Build history of the part. All positions in model axes, mm. A direction names the side the tool comes from. Coordinates: 2 decimals unless noted, no trailing zeros. Order: outer loops, then holes, each group sorted by start corner. A loop starts at its lowest first (then second) coordinate and runs counter-clockwise, first axis right, second up. Notation, with made-up numbers: (12.25, -17.5) - (26.25, -17.5) arc R17 cw to (26.25, 3.5) - close; hole circle Ø7 at (39.25, -26.5). An arc over 180 degrees is marked (long way). One line per item, written item: value.
from build123d import *

# Parameters (mm, degrees)
F1_START = -5
F1_DEPTH = 5
F2_DEPTH = 5
F3_DEPTH = 10
F4_DEPTH = 5
F5_DEPTH = 5


# Not quite as in the source:
# - after a boolean that leaves OpenCascade's solid faulty, fix() repairs it
# - a feature names something its author has since deleted; it is built from what else it names


with BuildPart() as f1:
    # F0 (on Top) → F1 (new body)
    with BuildSketch(Plane.XY.offset(F1_START)):
        with BuildLine():
            Line((0, 12), (-48.538644398, 12))
            Line((-48.538644398, 12), (-53.6749476013, 12))
            Line((-53.6749476013, 12), (-57.7667724561, 12))
            Line((-57.7667724561, 12), (-67.9485099174, 12))
            ThreePointArc((-67.9485099174, 12), (-68.6421053306, 7.0186448683), (-68.9710084021, 2))
            Line((-68.9710084021, 2), (0, 2))
            Line((0, 2), (0, 12))
        make_face()
        with BuildLine():
            Line((0, -7), (0, -2))
            Line((0, -2), (-68.9710084021, -2))
            ThreePointArc((-68.9710084021, -2), (-68.8529103806, -4.5029692558), (-68.6440092069, -7))
            Line((-68.6440092069, -7), (-58.5832740635, -7))
            Line((-58.5832740635, -7), (-54.5527267879, -7))
            Line((-54.5527267879, -7), (-49.5075751779, -7))
            Line((-49.5075751779, -7), (0, -7))
        make_face()
        with BuildLine():
            Line((68.9710084021, -2), (0, -2))
            Line((0, -2), (0, -7))
            Line((0, -7), (49.5075751779, -7))
            Line((49.5075751779, -7), (54.5527267879, -7))
            Line((54.5527267879, -7), (58.5832740635, -7))
            Line((58.5832740635, -7), (68.6440092069, -7))
            ThreePointArc((68.6440092069, -7), (68.8529103806, -4.5029692558), (68.9710084021, -2))
        make_face()
        with BuildLine():
            Line((68.9710084021, 2), (0, 2))
            Line((0, 2), (0, 0))
            Line((0, 0), (0, -2))
            Line((0, -2), (68.9710084021, -2))
            ThreePointArc((68.9710084021, -2), (68.9927517198, -1.0001050586), (69, 0))
            ThreePointArc((69, 0), (68.9927517198, 1.0001050586), (68.9710084021, 2))
        make_face()
        with BuildLine():
            Line((53.6749476013, 12), (48.538644398, 12))
            Line((48.538644398, 12), (0, 12))
            Line((0, 12), (0, 2))
            Line((0, 2), (68.9710084021, 2))
            ThreePointArc((68.9710084021, 2), (68.6421053306, 7.0186448683), (67.9485099174, 12))
            Line((67.9485099174, 12), (57.7667724561, 12))
            Line((57.7667724561, 12), (53.6749476013, 12))
        make_face()
        with BuildLine():
            Line((0, 0), (0, 2))
            Line((0, 2), (-68.9710084021, 2))
            ThreePointArc((-68.9710084021, 2), (-69, 0), (-68.9710084021, -2))
            Line((-68.9710084021, -2), (0, -2))
            Line((0, -2), (0, 0))
        make_face()
    extrude(amount=-F1_DEPTH)

    # F0 (on Top) → F2 (join)
    with BuildSketch(Plane.XY):
        with BuildLine():
            Line((0, -7), (0, -2))
            Line((0, -2), (-68.9710084021, -2))
            ThreePointArc((-68.9710084021, -2), (-68.8529103806, -4.5029692558), (-68.6440092069, -7))
            Line((-68.6440092069, -7), (-58.5832740635, -7))
            Line((-58.5832740635, -7), (-54.5527267879, -7))
            Line((-54.5527267879, -7), (-49.5075751779, -7))
            Line((-49.5075751779, -7), (0, -7))
        make_face()
        with BuildLine():
            Line((0, 12), (-48.538644398, 12))
            Line((-48.538644398, 12), (-53.6749476013, 12))
            Line((-53.6749476013, 12), (-57.7667724561, 12))
            Line((-57.7667724561, 12), (-67.9485099174, 12))
            ThreePointArc((-67.9485099174, 12), (-68.6421053306, 7.0186448683), (-68.9710084021, 2))
            Line((-68.9710084021, 2), (0, 2))
            Line((0, 2), (0, 12))
        make_face()
        with BuildLine():
            Line((53.6749476013, 12), (48.538644398, 12))
            Line((48.538644398, 12), (0, 12))
            Line((0, 12), (0, 2))
            Line((0, 2), (68.9710084021, 2))
            ThreePointArc((68.9710084021, 2), (68.6421053306, 7.0186448683), (67.9485099174, 12))
            Line((67.9485099174, 12), (57.7667724561, 12))
            Line((57.7667724561, 12), (53.6749476013, 12))
        make_face()
        with BuildLine():
            Line((68.9710084021, -2), (0, -2))
            Line((0, -2), (0, -7))
            Line((0, -7), (49.5075751779, -7))
            Line((49.5075751779, -7), (54.5527267879, -7))
            Line((54.5527267879, -7), (58.5832740635, -7))
            Line((58.5832740635, -7), (68.6440092069, -7))
            ThreePointArc((68.6440092069, -7), (68.8529103806, -4.5029692558), (68.9710084021, -2))
        make_face()
    extrude(amount=-F2_DEPTH)

    # F0 (on Top) → F3 (join)
    with BuildSketch(Plane.XY):
        with BuildLine():
            ThreePointArc((-57.7667724561, 12), (0, 59), (57.7667724561, 12))
            Line((57.7667724561, 12), (67.9485099174, 12))
            ThreePointArc((67.9485099174, 12), (0, 69), (-67.9485099174, 12))
            Line((-67.9485099174, 12), (-57.7667724561, 12))
        make_face()
        with BuildLine():
            Line((-58.5832740635, -7), (-68.6440092069, -7))
            ThreePointArc((-68.6440092069, -7), (0, -69), (68.6440092069, -7))
            Line((68.6440092069, -7), (58.5832740635, -7))
            ThreePointArc((58.5832740635, -7), (0, -59), (-58.5832740635, -7))
        make_face()
    extrude(amount=-F3_DEPTH)

    # F0 (on Top) → F4 (join)
    with BuildSketch(Plane.XY):
        with BuildLine():
            Line((54.5527267879, -7), (49.5075751779, -7))
            ThreePointArc((49.5075751779, -7), (0, -50), (-49.5075751779, -7))
            Line((-49.5075751779, -7), (-54.5527267879, -7))
            ThreePointArc((-54.5527267879, -7), (0, -55), (54.5527267879, -7))
        make_face()
        with BuildLine():
            ThreePointArc((-48.538644398, 12), (0, 50), (48.538644398, 12))
            Line((48.538644398, 12), (53.6749476013, 12))
            ThreePointArc((53.6749476013, 12), (0, 55), (-53.6749476013, 12))
            Line((-53.6749476013, 12), (-48.538644398, 12))
        make_face()
        with BuildLine():
            ThreePointArc((-53.6749476013, 12), (0, 55), (53.6749476013, 12))
            Line((53.6749476013, 12), (57.7667724561, 12))
            ThreePointArc((57.7667724561, 12), (0, 59), (-57.7667724561, 12))
            Line((-57.7667724561, 12), (-53.6749476013, 12))
        make_face()
        with BuildLine():
            Line((-54.5527267879, -7), (-58.5832740635, -7))
            ThreePointArc((-58.5832740635, -7), (0, -59), (58.5832740635, -7))
            Line((58.5832740635, -7), (54.5527267879, -7))
            ThreePointArc((54.5527267879, -7), (0, -55), (-54.5527267879, -7))
        make_face()
    extrude(amount=-F4_DEPTH)

    # F0 (on Top) → F5 (join)
    with BuildSketch(Plane.XY):
        with BuildLine():
            ThreePointArc((-57.7667724561, 12), (0, 59), (57.7667724561, 12))
            Line((57.7667724561, 12), (67.9485099174, 12))
            ThreePointArc((67.9485099174, 12), (0, 69), (-67.9485099174, 12))
            Line((-67.9485099174, 12), (-57.7667724561, 12))
        make_face()
        with BuildLine():
            ThreePointArc((-48.538644398, 12), (0, 50), (48.538644398, 12))
            Line((48.538644398, 12), (53.6749476013, 12))
            ThreePointArc((53.6749476013, 12), (0, 55), (-53.6749476013, 12))
            Line((-53.6749476013, 12), (-48.538644398, 12))
        make_face()
        with BuildLine():
            Line((-58.5832740635, -7), (-68.6440092069, -7))
            ThreePointArc((-68.6440092069, -7), (0, -69), (68.6440092069, -7))
            Line((68.6440092069, -7), (58.5832740635, -7))
            ThreePointArc((58.5832740635, -7), (0, -59), (-58.5832740635, -7))
        make_face()
        with BuildLine():
            Line((54.5527267879, -7), (49.5075751779, -7))
            ThreePointArc((49.5075751779, -7), (0, -50), (-49.5075751779, -7))
            Line((-49.5075751779, -7), (-54.5527267879, -7))
            ThreePointArc((-54.5527267879, -7), (0, -55), (54.5527267879, -7))
        make_face()
    extrude(amount=F5_DEPTH)

    add(f1.part.fix(), mode=Mode.REPLACE)


solid = f1.part
1. Probe line 1 along X through (y, z) = (45.5, 0.25); line 2 along X through (y, z) = (29.5, 2.25); line 3 along Y through (x, z) = (10, 4.25). List the from-to ranges inside material, lowest first.
Values found:
line 1: x = -51.87 to -37.56, -30.9 to -20.73, 20.73 to 30.9, 37.56 to 51.87
line 2: x = -62.38 to -51.1, -46.42 to -40.37, 40.37 to 46.42, 51.1 to 62.38
line 3: y = -68.27 to -58.15, -54.08 to -48.99, 48.99 to 54.08, 58.15 to 68.27
2. 3-axis set-ups, long thin cutter, end or side, ignore diameter. For faces 1 (the face through (-0.3, -50.4, 5)), 2 (the face through (-0.3, -50.2, -5)), 3 (the face through (-1.13, 58.99, 2.46)), 4 (the face through (-51, 12, 2)): which of +Z, -Z, +X, -X, +Y, -Y reach the whole face in a straight line?
Values found:
face 1: +Z, +X, -X, +Y, -Y
face 2: -Z
face 3: +Z
face 4: +Z, +X, -X
3. Band-saw the part on D-D, the plane y = -45. Give the cut face in (x, z).
Values found:
outline: (-52.31, -10) - (-38.16, -10) - (-38.16, -5) - (-21.79, -5) - (-21.79, 5) - (-31.62, 5) - (-31.62, 0) - (-38.16, 0) - (-38.16, 5) - (-52.31, 5) - close; (21.79, -5) - (38.16, -5) - (38.16, -10) - (52.31, -10) - (52.31, 5) - (38.16, 5) - (38.16, 0) - (31.62, 0) - (31.62, 5) - (21.79, 5) - close
4. Band-saw the part on C-C, the plane x = -10.5. Give the cut face in (y, z).
Values found:
outline: (-68.2, -10) - (-58.06, -10) - (-58.06, -5) - (-48.89, -5) - (-48.89, 5) - (-53.99, 5) - (-53.99, 0) - (-58.06, 0) - (-58.06, 5) - (-68.2, 5) - close; (-7, -10) - (12, -10) - (12, 0) - (2, 0) - (2, -5) - (-2, -5) - (-2, 0) - (-7, 0) - close; (48.89, -5) - (58.06, -5) - (58.06, -10) - (68.2, -10) - (68.2, 5) - (58.06, 5) - (58.06, 0) - (53.99, 0) - (53.99, 5) - (48.89, 5) - close
5. Band-saw the part on A-A, the plane z = -2.5. Give the cut face in (x, y).
Values found:
outline: (-68.97, -2) arc R69 ccw to (68.97, -2) - close; (-68.97, 2) - (68.97, 2) arc R69 ccw to start; hole (-49.51, -7) arc R50 ccw to (49.51, -7) - close; hole (-48.54, 12) - (48.54, 12) arc R50 ccw to start
6. Flat gauge pins, fed straight in: P1, Ø4, axis at x = -52.5, z = -4.5, coming from the -Y side; P2, Ø12, axis at x = -21.5, y = 12.5, coming from the -Z side; P3, Ø5.5, axis at x = 63.5, z = 3, coming from the +Y side; P4, Ø3, axis at x = -24.5, z = -4, coming from the -Y side. Where does each tip first touch, or does it go through?
Values found:
P1: stops at y = -47.02
P2: stops at z = -10
P3: stops at y = 32.72
P4: stops at y = -65.05
7. Two-plate mould, pull along X, no slides. Class faces 5 (the face through (-1.11, -54.99, 2.46)), 6 (the face through (-5, 60, 5)): pulls with the +X half, pulls with the -X half, needs draft (parallel to the pull), parting line crosses it, or undercut.
Values found:
face 5: undercut
face 6: needs draft
8. Band-saw the part on B-B, the plane y = -19. Give the cut face in (x, z), and give its area (3 significant figures).
Values found:
outline: (-66.33, -10) - (-55.86, -10) - (-55.86, -5) - (-46.25, -5) - (-46.25, 5) - (-51.61, 5) - (-51.61, 0) - (-55.86, 0) - (-55.86, 5) - (-66.33, 5) - close; (46.25, -5) - (55.86, -5) - (55.86, -10) - (66.33, -10) - (66.33, 5) - (55.86, 5) - (55.86, 0) - (51.61, 0) - (51.61, 5) - (46.25, 5) - close
area: 464 mm2
